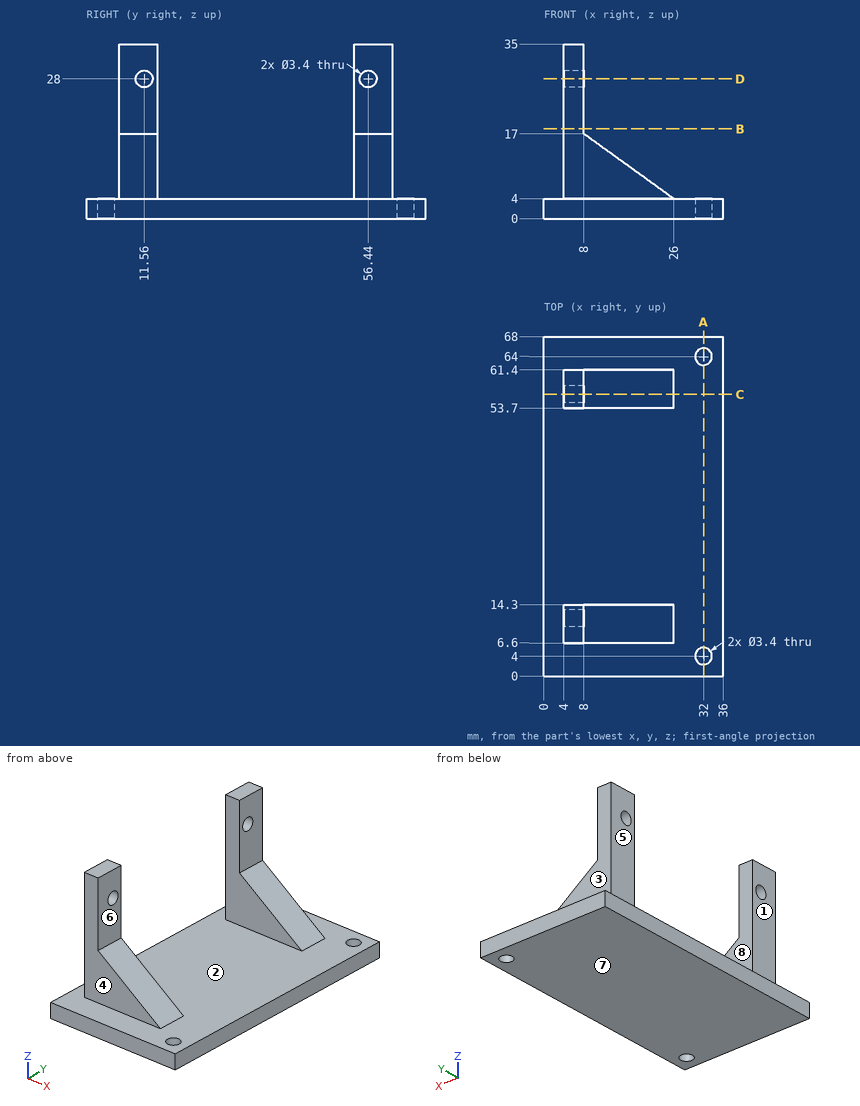
Design review of the part shown in the three views and the two pictorial views. Dimensions are in mm from the part's minimum x, y and z. A direction names the side the tool comes from. Round coordinates to 2 decimals unless told otherwise and drop trailing zeros. Order: outer loops, then holes, each group sorted by start corner. A loop starts at its lowest first (then second) coordinate and runs counter-clockwise, first axis right, second up.
Q1. Mouldability with a two-part tool opening along Y and no side actions: class the marked faces 1, 2, 3 and 4 as pulls with the +Y half, pulls with the -Y half, needs draft (parallel to the pull), parting line crosses it, or undercut.
Findings below:
face 1: needs draft
face 2: undercut
face 3: pulls with the +Y half
face 4: pulls with the -Y half
Q2. We need section A-A, the plane x = 32. Give the boundary of the cut face in (y, z).
Findings below:
outline: (0, 0) - (2.3, 0) - (2.3, 4) - (0, 4) - close; (5.7, 0) - (62.3, 0) - (62.3, 4) - (5.7, 4) - close; (65.7, 0) - (68, 0) - (68, 4) - (65.7, 4) - close
Q3. We need section B-B, the plane z = 18. Give the boundary of the cut face in (x, y), plus the area to 3 significant figures.
Findings below:
outline: (4, 6.6) - (8, 6.6) - (8, 14.3) - (4, 14.3) - close; (4, 53.7) - (8, 53.7) - (8, 61.4) - (4, 61.4) - close
area: 61.6 mm2
Q4. We need section C-C, the plane y = 56.44. Give the boundary of the cut face in (x, z).
Findings below:
outline: (0, 0) - (36, 0) - (36, 4) - (26, 4) - (8, 17) - (8, 26.3) - (4, 26.3) - (4, 4) - (0, 4) - close; (4, 29.7) - (8, 29.7) - (8, 35) - (4, 35) - close
Q5. Machinability: for the marked faces 5, 6, 7 and 8, which of the approach directions +Z, -Z, +X, -X, +Y, -Y give a long, thin tool a straight path to every point of the face, cutting with its end or side? Answer none if there is none.
Findings below:
face 5: +Z, -X, +Y, -Y
face 6: +Z, +X, +Y, -Y
face 7: -Z, +X, -X, +Y, -Y
face 8: +Z, +X, -X
Q6. We need section D-D, the plane z = 28. Give the boundary of the cut face in (x, y).
Findings below:
outline: (4, 6.6) - (8, 6.6) - (8, 9.86) - (4, 9.86) - close; (4, 13.26) - (8, 13.26) - (8, 14.3) - (4, 14.3) - close; (4, 53.7) - (8, 53.7) - (8, 54.74) - (4, 54.74) - close; (4, 58.14) - (8, 58.14) - (8, 61.4) - (4, 61.4) - close
Q7. Wall thickness on line 1 (Y direction, x = 6.25, z = 28); line 2 (X direction, y = 4, z = 1); line 3 (Y direction, x = 6.5, z = 8.5): over which ranges is each line inside the solid? List them lowest first.
Findings below:
line 1: y = 6.6 to 9.86, 13.26 to 14.3, 53.7 to 54.74, 58.14 to 61.4
line 2: x = 0 to 30.3, 33.7 to 36
line 3: y = 6.6 to 14.3, 53.7 to 61.4
Q8. Insertion check: P1, Ø8.5, axis at y = 10.5, z = 27, coming from the +X side; P2, Ø2.5, axis at y = 56.44, z = 28, coming from the -X side; P3, Ø8, axis at x = 4.5, y = 13.5, coming from the -Z side; P4, Ø18, axis at x = 20, y = 50.5, coming from the +Z side. Each pin has a flat end and moves straight along its axis. Give the tip position at first contact, or say it passes through.
Findings below:
P1: stops at x = 8
P2: passes through
P3: stops at z = 0
P4: stops at z = 14.41
